Geometry: final body of the model. Coordinates: model frame, mm. Face numbers are marked on the shaded views. A direction names the side the tool comes from. Coordinates: 2 decimals unless noted, no trailing zeros. Order: outer loops, then holes, each group sorted by start corner. A loop starts at its lowest first (then second) coordinate and runs counter-clockwise, first axis right, second up. Notation, with made-up numbers: (4.25, -37) - (43.25, -37) arc R16 cw to (43.25, -20) - close; hole circle Ø5 at (77, 85.5). An arc over 180 degrees is marked (long way). Use a Markdown table: item, result. Add a question column.
```python
from build123d import *

# Parameters (mm, degrees)
F2_R           = 1.25
F3_DEPTH       = 50.001
F4_R           = 2
F5_DEPTH       = 35
F7_D           = 8
F7_DEPTH       = 10
F7_CSINK_D     = 10
F7_CSINK_ANGLE = 90
F7_TIP         = 2.4034424761


with BuildPart() as f1:
    # F0 (on Front) → F1 (revolve)
    with BuildSketch(Plane.XZ):
        Polygon((6.2365774143, -10), (10, 0), (0, 0), (0, -50), (3.15, -50), (3.15, -40), (3.15, -30), (10, -30), (10, -10), align=None)
        with BuildLine():
            add(Edge.make_bspline(
                [(10, -30), (7.4056518976, -31.2777532916), (6.0791644046, -31.9480016), (3.9945104258, -34.715284016), (3.61089129, -36.7225967348), (3.15, -40)],
                knots=[0, 0, 0, 0, 0.3551625171, 0.6094131259, 1, 1, 1, 1], degree=3))
            Line((10, -30), (3.15, -30))
            Line((3.15, -30), (3.15, -40))
        make_face()
    revolve(axis=Axis((0, 0, -25), (0, 0, 1)))

    # F2 (on face) → F3 (cut, through all)
    with BuildSketch(Plane(origin=(0, 0, -50), x_dir=(1, 0, 0), z_dir=(0, 0, -1))):
        Circle(F2_R)
    extrude(amount=-F3_DEPTH, mode=Mode.SUBTRACT)

    # F4 (on face) → F5 (cut)
    with BuildSketch(Plane(origin=(0, 0, -50), x_dir=(1, 0, 0), z_dir=(0, 0, -1))):
        Circle(F4_R)
    extrude(amount=F5_DEPTH, mode=Mode.SUBTRACT)

    # F7
    with Locations(Plane.XY):
        with Locations((0, 0)):
            CounterSinkHole(F7_D / 2, F7_CSINK_D / 2, depth=F7_DEPTH, counter_sink_angle=F7_CSINK_ANGLE)
            with Locations((0, 0, -(F7_DEPTH + F7_TIP / 2))):  # 118° drill point
                Cone(0, F7_D / 2, F7_TIP, mode=Mode.SUBTRACT)


solid = f1.part
```
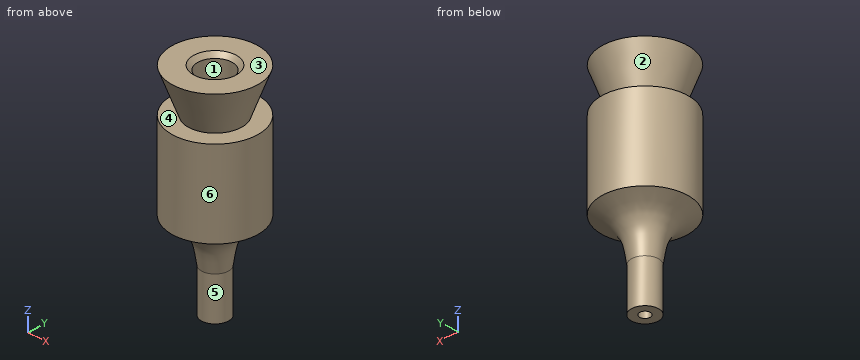
1) First-contact query: pin 1 (5 mm diameter, centred on y = -7.5, z = -12, fed in from +X); pin 2 (6 mm diameter, centred on x = -0.5, y = 1.5, fed in from +Z); pin 3 (12 mm diameter, centred on x = -1, z = -24.5, fed in from +Y); pin 4 (3 mm diameter, centred on x = 0, y = 0, fed in from +Z). Flat tips, straight axial feed; report the tip coordinate or a pass-through.
2) Line query: line 1 (Y direction, x = 0, z = -23); line 2 (Y direction, x = 0, z = -3.75); line 3 (X direction, y = 0, z = -4). Output: solid intervals per line, ascending. Write a range as from..to.
3) Access query for the marked faces 4, 5 and 6. Directions: +Z, -Z, +X, -X, +Y, -Y. A direction counts if a zero-diameter tool reaches every point of the face in a straight line with its end or side. Return the directions, or none.
4) Draft query along Y for the marked faces 1, 2 and 3. Return one class per face: released by +Y, released by -Y, zero draft, split by the parting line, or undercut.
5) Section query B-B (z = -26.5). Return the cut outline in (x, y).
6) Section query A-A (z = -43). Return the cut outline in (x, y), and give its area (3 significant figures).
From the geometry:
| question | item | result |
|---|---|---|
| 1 | pin 1 | stops at x = 8.66 |
| 1 | pin 2 | stops at z = -0.42 |
| 1 | pin 3 | stops at y = 10 |
| 1 | pin 4 | stops at z = -11.5 |
| 2 | line 1 | y = -10..-1.25, 1.25..10 |
| 2 | line 2 | y = -8.59..-4, 4..8.59 |
| 2 | line 3 | x = -8.49..-4, 4..8.49 |
| 3 | face 4 | none |
| 3 | face 5 | -Z |
| 3 | face 6 | +Z, -Z |
| 4 | face 1 | undercut |
| 4 | face 2 | split by the parting line |
| 4 | face 3 | zero draft |
| 5 | outline | circle Ø20 at (0, 0); hole circle Ø2.5 at (0, 0) |
| 6 | outline | circle Ø6.3 at (0, 0); hole circle Ø2.5 at (0, 0) |
| 6 | area | 26.3 mm^2 |
